Design review of the part built by this model. Coordinates are the model's own, in mm. Face numbers are marked on the shaded views. A direction names the side the tool comes from. Coordinates: 2 decimals unless noted, no trailing zeros. Loops run counter-clockwise (first coordinate to the right, second up) from the corner with the lowest first, then second, coordinate; pieces in that order, holes last. Notation, with made-up numbers: (37.25, -28) -> (84.25, -28) arc R5 ccw to (84.25, -22) -> close; hole circle Ø10 at (64.25, 28). An arc over 180 degrees is marked (long way). Use CSV: the item, a comma, the result in double quotes.
```python
from build123d import *

# Parameters (mm, degrees)
BOSS_EXTRU_1_START      = 80
BOSS_EXTRU_1_DEPTH      = 100
ENL_V_START             = -80
ESQUISSE3_W             = 100
ESQUISSE3_H             = 16
ENL_V_MAT_EXTRU_1_DEPTH = 80
CONG_4_R                = 11
ESQUISSE4_R             = 20
ENL_V_MAT_EXTRU_2_DEPTH = 131.989866835


with BuildPart() as part:
    # Esquisse1 → Boss.-Extru.1 (new body)
    with BuildSketch(Plane.XY.offset(BOSS_EXTRU_1_START)):
        with BuildLine():
            Line((38.785545077, 40.614050057), (-40.651735145, 40.614050057))
            add(Edge.make_bspline(
                [(-40.651735145, 40.614050057), (-42.314401042, 40.614050057), (-43.949970441, 40.454492538), (-46.364281177, 39.985249726), (-47.162496652, 39.790237743), (-48.745517159, 39.321246489), (-49.533460665, 39.045648859), (-51.828661424, 38.115479858), (-53.281442172, 37.355862098), (-55.345438246, 36.008719052), (-56.014108587, 35.524812991), (-57.311227091, 34.484460801), (-57.928932966, 33.936606502), (-59.691288641, 32.213512357), (-60.746535217, 30.959092716), (-62.145716067, 28.915215354), (-62.582595679, 28.203507769), (-63.374918425, 26.755312757), (-63.732785576, 26.015863677), (-64.373256555, 24.506793589), (-64.65585931, 23.737172152), (-65.144921869, 22.167404719), (-65.351725199, 21.365590427), (-65.850986238, 18.923189743), (-66.017764036, 17.277412601), (-66.017764036, 15.614050057)],
                knots=[0, 0, 0, 0, 0.125, 0.125, 0.1875, 0.1875, 0.25, 0.25, 0.375, 0.375, 0.4375, 0.4375, 0.5, 0.5, 0.625, 0.625, 0.6875, 0.6875, 0.75, 0.75, 0.8125, 0.8125, 0.875, 0.875, 1, 1, 1, 1], degree=3))
            Line((-66.017764036, 15.614050057), (-66.017764036, -14.385949943))
            add(Edge.make_bspline(
                [(-66.017764036, -14.385949943), (-66.017764036, -16.048876138), (-65.851094207, -17.683331778), (-65.361702976, -20.094123219), (-65.158373409, -20.890853543), (-64.669502924, -22.47027084), (-64.382985964, -23.253871687), (-63.418861279, -25.531148199), (-62.632909001, -26.969986123), (-61.47342948, -28.670438694), (-61.23260127, -29.005579947), (-60.732801819, -29.665809665), (-60.473222797, -29.991558275), (-59.675187681, -30.943569432), (-59.115575096, -31.547471943), (-57.356561849, -33.269755718), (-56.077742546, -34.299557378), (-54.343422936, -35.435349924), (-53.989857778, -35.654684562), (-53.276724993, -36.073359456), (-52.916218587, -36.273332214), (-51.823086229, -36.845648188), (-50.334662142, -37.535258588), (-48.785246215, -38.079902579), (-47.20487869, -38.550980299), (-46.395575711, -38.750272405), (-43.957668722, -39.226451984), (-42.313993676, -39.385949943), (-40.651735145, -39.385949943)],
                knots=[0, 0, 0, 0, 0.125, 0.125, 0.1875, 0.1875, 0.25, 0.25, 0.375, 0.375, 0.40625, 0.40625, 0.4375, 0.4375, 0.5, 0.5, 0.625, 0.625, 0.65625, 0.65625, 0.6875, 0.6875, 0.75, 0.8125, 0.8125, 0.875, 0.875, 1, 1, 1, 1], degree=3))
            Line((-40.651735145, -39.385949943), (38.785545077, -39.385949943))
            add(Edge.make_bspline(
                [(38.785545077, -39.385949943), (40.442664026, -39.385949943), (42.072477718, -39.225354876), (44.477877986, -38.753201256), (45.273076472, -38.556989578), (46.849967737, -38.085132809), (47.634388323, -37.807976207), (49.917807144, -36.873298226), (51.362544447, -36.110292076), (53.414281907, -34.757655279), (54.079899229, -34.270978942), (55.366402243, -33.228584654), (55.97873177, -32.679974918), (57.725866743, -30.954489737), (58.771668074, -29.698711403), (60.157750527, -27.653150155), (60.589614996, -26.942198814), (61.372344654, -25.496840481), (62.079494348, -24.020824341), (62.637956251, -22.484495371), (63.121147278, -20.91763397), (63.325643893, -20.116192861), (63.817740886, -17.683150497), (63.982235964, -16.043440912), (63.982235964, -14.385949943)],
                knots=[0, 0, 0, 0, 0.125, 0.125, 0.1875, 0.1875, 0.25, 0.25, 0.375, 0.375, 0.4375, 0.4375, 0.5, 0.5, 0.625, 0.625, 0.6875, 0.6875, 0.75, 0.8125, 0.8125, 0.875, 0.875, 1, 1, 1, 1], degree=3))
            Line((63.982235964, -14.385949943), (63.982235964, 15.614050057))
            add(Edge.make_bspline(
                [(63.982235964, 15.614050057), (63.982235964, 17.271310828), (63.817806647, 18.900524173), (63.334809815, 21.304028451), (63.134123418, 22.098426882), (62.65157662, 23.673377539), (62.368548411, 24.455463484), (61.415616974, 26.729252988), (60.63846114, 28.166500735), (59.491466105, 29.865784629), (59.253210251, 30.200733657), (58.758705823, 30.860661599), (58.501710157, 31.186502863), (57.710451504, 32.140097193), (57.155472753, 32.745084226), (55.410698291, 34.47070563), (54.141818247, 35.502843902), (52.420489637, 36.641694741), (52.068783545, 36.862138502), (51.359150828, 37.2830162), (51.00041085, 37.484029901), (49.912631681, 38.059303906), (48.431489045, 38.75242056), (46.889689036, 39.299828689), (45.317129339, 39.773347224), (44.511672713, 39.973796439), (42.081029739, 40.453478808), (40.442443449, 40.614050057), (38.785545077, 40.614050057)],
                knots=[0, 0, 0, 0, 0.125, 0.125, 0.1875, 0.1875, 0.25, 0.25, 0.375, 0.375, 0.40625, 0.40625, 0.4375, 0.4375, 0.5, 0.5, 0.625, 0.625, 0.65625, 0.65625, 0.6875, 0.6875, 0.75, 0.8125, 0.8125, 0.875, 0.875, 1, 1, 1, 1], degree=3))
        make_face()
    extrude(amount=-BOSS_EXTRU_1_DEPTH)

    # Esquisse3 → Enlèv. mat.-Extru.1 (cut)
    with BuildSketch(Plane(origin=(0, 0, -20), x_dir=(-1, 0, 0), z_dir=(0, 0, -1)).offset(ENL_V_START)):
        with Locations((0.484895913, -0.273885368)):
            Rectangle(ESQUISSE3_W, ESQUISSE3_H)
    extrude(amount=ENL_V_MAT_EXTRU_1_DEPTH, mode=Mode.SUBTRACT)

    # Congé4
    cong_4_edges = [part.edges().sort_by_distance(p)[0] for p in [
        (49.515104087, -0.273885368, 60),
        (-50.484895913, -0.273885368, 60),
    ]]
    fillet(cong_4_edges, radius=CONG_4_R)

    # Esquisse4 → Enlèv. mat.-Extru.2 (cut, through all)
    with BuildSketch(Plane.XZ.offset(39.385949943)):
        with Locations((0, 20)):
            Circle(ESQUISSE4_R)
    extrude(amount=-ENL_V_MAT_EXTRU_2_DEPTH, mode=Mode.SUBTRACT)


solid = part.part
```
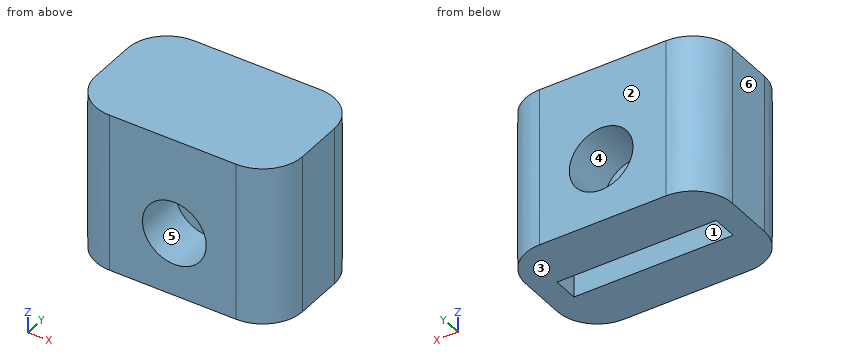
Item 1: Add section B-B (y = 11.5). Give the boundary of the cut face in (x, z).
Checked values:
outline,"(-66.02, -20) -> (63.98, -20) -> (63.98, 80) -> (-66.02, 80) -> close; hole circle Ø40 at (0, 20)"
Item 2: Machinability: for the marked faces 1 and 2, which of the approach directions +Z, -Z, +X, -X, +Y, -Y give a long, thin tool a straight path to every point of the face, cutting with its end or side? Answer none if there is none.
Checked values:
face 1,"-Z"
face 2,"+Z, -Z, +X, -X, +Y"
Item 3: Draft analysis for pull direction Z (two halves, no side actions). For the marked faces 3, 4, 5 and 6, state which applies: pulls with the +Z half, pulls with the -Z half, needs draft (parallel to the pull), parting line crosses it, or undercut.
Checked values:
face 3,"pulls with the -Z half"
face 4,"undercut"
face 5,"undercut"
face 6,"needs draft"
Item 4: To check wall thickness, follow line 1 along Y through (x, z) = (38, 54.5); line 2 along Z through (x, y) = (0, 20); line 3 along Z through (x, y) = (30.5, 3.5). State the ranges of each line that lie inside material, in increasing order.
Checked values:
line 1,"-39.39 to -8.27, 7.73 to 40.61"
line 2,"-20 to 0, 40 to 80"
line 3,"60 to 80"
Item 5: Add section A-A (x = 0). Give the boundary of the cut face in (y, z), then the cut area to 3 significant figures.
Checked values:
outline,"(-39.39, -20) -> (-8.27, -20) -> (-8.27, 0) -> (-39.39, 0) -> close; (-39.39, 40) -> (-8.27, 40) -> (-8.27, 60) -> (7.73, 60) -> (7.73, 40) -> (40.61, 40) -> (40.61, 80) -> (-39.39, 80) -> close; (7.73, -20) -> (40.61, -20) -> (40.61, 0) -> (7.73, 0) -> close"
area,"4,160 mm^2"
Item 6: Clearance check with flat-ended pins moving along their axes: pin 1 (2 mm diameter, centred on y = -31, z = 8, fed in from +X); pin 2 (24 mm diameter, centred on x = 0, z = 20, fed in from -Y); pin 3 (8 mm diameter, centred on x = 11, y = -3, fed in from -Z); pin 4 (1.5 mm diameter, centred on y = -16, z = 15, fed in from +X). State where each tip first meets the part, or that it passes through.
Checked values:
pin 1,"x = 58.46"
pin 2,"through"
pin 3,"z = 60"
pin 4,"x = 63.97"
Item 7: Add section D-D (x = -17.5). Give the boundary of the cut face in (y, z), then the cut area to 3 significant figures.
Checked values:
outline,"(-39.39, -20) -> (-8.27, -20) -> (-8.27, 10.32) -> (-39.39, 10.32) -> close; (-39.39, 29.68) -> (-8.27, 29.68) -> (-8.27, 60) -> (7.73, 60) -> (7.73, 29.68) -> (40.61, 29.68) -> (40.61, 80) -> (-39.39, 80) -> close; (7.73, -20) -> (40.61, -20) -> (40.61, 10.32) -> (7.73, 10.32) -> close"
area,"5,480 mm^2"
Item 8: Add section C-C (x = 23). Give the boundary of the cut face in (y, z), then the cut area to 3 significant figures.
Checked values:
outline,"(-39.39, -20) -> (-8.27, -20) -> (-8.27, 60) -> (7.73, 60) -> (7.73, -20) -> (40.61, -20) -> (40.61, 80) -> (-39.39, 80) -> close"
area,"6,720 mm^2"
